```python
from build123d import *

# Parameters (mm, degrees)
SKETCH1_W           = 6.1
SKETCH1_H           = 9
BOSS_EXTRUDE1_DEPTH = 9.29
SKETCH3_R           = 2
CUT_EXTRUDE2_DEPTH  = 12.990166805
SKETCH4_W           = 6.1
SKETCH4_H           = 9
BOSS_EXTRUDE2_DEPTH = 196.7


with BuildPart() as part:
    # Sketch1 → Boss-Extrude1 (new body)
    with BuildSketch(Plane.XY):
        Rectangle(SKETCH1_W, SKETCH1_H)
    extrude(amount=BOSS_EXTRUDE1_DEPTH)

    # Sketch3 → Cut-Extrude2 (cut, through all)
    with BuildSketch(Plane(origin=(3.05, 0, 0), x_dir=(0, 0, -1), z_dir=(1, 0, 0))):
        with BuildLine():
            ThreePointArc((-4.5, 4.5), (-1.318019485, 3.181980515), (0, 0))
            Line((0, 0), (0, 4.5))
            Line((0, 4.5), (-4.5, 4.5))
        make_face()
        with BuildLine():
            ThreePointArc((0, 0), (-1.318019485, -3.181980515), (-4.5, -4.5))
            Line((-4.5, -4.5), (0, -4.5))
            Line((0, -4.5), (0, 0))
        make_face()
        with Locations((-4.8, 0)):
            Circle(SKETCH3_R)
    extrude(amount=-CUT_EXTRUDE2_DEPTH, mode=Mode.SUBTRACT)

    # Sketch4 → Boss-Extrude2 (add)
    with BuildSketch(Plane.XY.offset(9.29)):
        Rectangle(SKETCH4_W, SKETCH4_H)
    extrude(amount=BOSS_EXTRUDE2_DEPTH)


solid = part.part
```
The listing builds one solid part. Answer for the finished solid, in the listing's coordinates (mm). Round coordinates to 2 decimals unless told otherwise and drop trailing zeros.
1) Given P1, Ø5, axis at y = 0, z = 4.8, coming from the +X side, flat-ended and moving along its own axis, determine where the tip first touches the part or whether it passes through.
Outcome:
P1: stops at x = 3.05
2) For a pull along Z with two mould halves and no side action, classify faces 1 (the face through (0, 0, 205.99)), 2 (the face through (0.043, -0.766, 2.953)), 3 (the face through (3.05, 0, 102)) as released by +Z, released by -Z, zero draft, split by the parting line, or undercut.
Outcome:
face 1: released by +Z
face 2: undercut
face 3: zero draft
3) Consider line 1 (Y direction, x = -0.75, z = 4.8); line 2 (Z direction, x = -1.25, y = 1.75); line 3 (Z direction, x = 1.5, y = 3.75). Determine where each line is inside the solid, lowest interval first.
Outcome:
line 1: y = -4.5 to -2, 2 to 4.5
line 2: z = 0.35 to 3.83, 5.77 to 205.99
line 3: z = 2.01 to 205.99
